Solid Edge part; units mm, degrees
sketch "Sketch1" plane through (0, 0, 0) normal (0, 0, 1) x (1, 0, 0)
  line L0 (-10.0513, -24.5) -> (10.0513, -24.5)
  line L1 (10.0513, -24.5) -> (10.0513, 24.5)
  line L2 (10.0513, 24.5) -> (-10.0513, 24.5)
  line L3 (-10.0513, 24.5) -> (-10.0513, -24.5)
  circle A0 centre (0, 17.5) radius 2.6
  circle A1 centre (0, -17.5) radius 2.6
extrude "Protrusion1" add sketch "Sketch1" along normal blind 8
sketch "Sketch2" plane through (0, 0, 8) normal (0, 0, 1) x (1, 0, 0)
  circle A0 centre (0, 17.5) radius 4.5
  circle A1 centre (0, -17.5) radius 4.5
extrude "ExtrudedCutout_1" cut sketch "Sketch2" against normal blind 2
hole "Hole_1" at (-5.5, -24.5, 3) direction (0, 1, 0) diameter 2.459 depth 10 thread major 3 thread length 8
hole "Hole1" at (5.5, -24.5, 3) direction (0, 1, 0) diameter 2.459 depth 10 thread major 3 thread length 8
mirror "Mirror1" about plane through (0, 0, 0) normal (0, 1, 0) of "Hole_1", "Hole1"
Can you work these out from the model? Positions are in its coordinate system, mm. A direction names the side the tool comes from. Coordinates: 2 decimals unless noted, no trailing zeros. Write each loop counter-clockwise with the first axis right and the second up, starting at its lowest first coordinate (ties: lowest second). Pieces come first, ordered by that corner, then holes. Notation, with made-up numbers: M -37.5,-15.5 L -29.5,-15.5 A7 cw -29.5,-3.5 Z; hole C -11,18.5 d1. An arc over 180 degrees is marked long. Write item = value, one per line. Start each with the question number.
Q1. If we section it at D-D, the plane x = 5.5: Write out the boundary of the cut face in (y, z), then the cut area to 3 significant figures.
Q2. If I drill on L1, parallel to Y at x = 0, z = 7.05; L2, parallel to X at y = 22.25, z = 3; L3, parallel to Y at x = 2, z = 6.75, over which ranges is the centre line in solid material (lowest first)? Write a range as [from, to].
Q3. I'm going to push flat-ended pins straight in: pin 1 (8.5 mm diameter, centred on x = 0, y = -17.5, fed in from -Z); pin 2 (5.5 mm diameter, centred on x = 0, y = -17.5, fed in from +Z); pin 3 (0.7 mm diameter, centred on x = 6, z = 3.5, fed in from -Y); pin 4 (2 mm diameter, centred on x = 5.5, z = 3, fed in from +Y). Where does each tip first touch, or does it pass through?
Q4. Thinking about a two-plate mould opening in Z: for faces 1 (the face through (-0.1, -20.4, 6)), 2 (the face through (-6, -14.5, 3)), 3 (the face through (10.051, 0, 4)), 4 (the face through (5, 14.5, 3)), which applies, released by +Z, released by -Z, zero draft, split by the parting line, or undercut?
Q5. If we section it at C-C, the plane z = 3: Write out the boundary of the cut face in (x, y).
Q6. If we section it at A-A, the plane y = -17.5: Write out the boundary of the cut face in (x, z).
Q7. If we section it at B-B, the plane x = 0: Write out the boundary of the cut face in (y, z).
Q8. On a 3-axis mill with a long thin cutter (end or side, diameter ignored), from which of +Z, -Z, +X, -X, +Y, -Y can I reach the whole of each face in a straight line? I mean faces 5 (the face through (-6.59, 19.43, 2.43)), 6 (the face through (0, -24.5, 4)), 7 (the face through (-4.41, -19.43, 2.43)), 8 (the face through (-0.59, 21.96, 7.01)), 9 (the face through (-0.338, 14.922, 2.958)). Say none if no direction works.
Check sheet entries:
q1.outline = M -24.5,0 L 24.5,0 L 24.5,1.77 L 14.5,1.77 L 14.5,4.23 L 24.5,4.23 L 24.5,8 L -24.5,8 L -24.5,4.23 L -14.5,4.23 L -14.5,1.77 L -24.5,1.77 Z
q1.area = 343 mm²
q2.L1 = [-24.5, -22], [-13, 13], [22, 24.5]
q2.L2 = [-10.05, -6.73], [-4.27, 4.27], [6.73, 10.05]
q2.L3 = [-24.5, -21.53], [-13.47, 13.47], [21.53, 24.5]
q3.pin_1 = 0
q3.pin_2 = 6
q3.pin_3 = -14.5
q3.pin_4 = 14.5
q4.face_1 = released by +Z
q4.face_2 = undercut
q4.face_3 = zero draft
q4.face_4 = undercut
q5.outline = M -10.05,-24.5 L -6.73,-24.5 L -6.73,-14.5 L -4.27,-14.5 L -4.27,-24.5 L 4.27,-24.5 L 4.27,-14.5 L 6.73,-14.5 L 6.73,-24.5 L 10.05,-24.5 L 10.05,24.5 L 6.73,24.5 L 6.73,14.5 L 4.27,14.5 L 4.27,24.5 L -4.27,24.5 L -4.27,14.5 L -6.73,14.5 L -6.73,24.5 L -10.05,24.5 Z; hole C 0,-17.5 d5.2; hole C 0,17.5 d5.2
q6.outline = M -10.05,0 L -2.6,0 L -2.6,6 L -4.5,6 L -4.5,8 L -10.05,8 Z; M 2.6,0 L 10.05,0 L 10.05,8 L 4.5,8 L 4.5,6 L 2.6,6 Z; hole C -5.5,3 d2.46; hole C 5.5,3 d2.46
q7.outline = M -24.5,0 L -20.1,0 L -20.1,6 L -22,6 L -22,8 L -24.5,8 Z; M -14.9,0 L 14.9,0 L 14.9,6 L 13,6 L 13,8 L -13,8 L -13,6 L -14.9,6 Z; M 20.1,0 L 24.5,0 L 24.5,8 L 22,8 L 22,6 L 20.1,6 Z
q8.face_5 = +Y
q8.face_6 = +Z, -Z, +X, -X, -Y
q8.face_7 = -Y
q8.face_8 = +Z
q8.face_9 = +Z, -Z
